Part model, mm, in its own coordinate system. Face numbers are marked on the shaded views. A direction names the side the tool comes from. Round coordinates to 2 decimals unless told otherwise and drop trailing zeros. Loops run counter-clockwise (first coordinate to the right, second up) from the corner with the lowest first, then second, coordinate; pieces in that order, holes last. Notation, with made-up numbers: M 56,54.25 L 72,54.25 A21 cw 72,92.25 Z; hole C 89,34 d2. An arc over 180 degrees is marked long. Put each result on its own line as item: value. Start each with the question number.
1) Drop a flat-ended pin along its axis: pin 1 Ø10 at (x, y) = (82, -842) entering from -Z. Give the stop position or say it passes through.
2) Slice it at C-C on z = 17. Give the cut face in (x, y).
3) Probe line 1 along X through (y, z) = (-778, 1.15); line 2 along X through (y, z) = (-776, 12); line 3 along Z through (x, y) = (9.5, -523.5). List the from-to ranges inside material, lowest first.
4) Pull direction X, two halves, no side cores. Call the marked faces 3 and 4: +X half, -X half, draft (parallel to the pull), parting line (faces both ways), or undercut.
5) Slice it at A-A on y = -115. Give the cut face in (x, z), then the cut area to 3 significant figures.
6) Slice it at B-B on x = 50. Give the cut face in (y, z).
7) Which spindle directions (+Z, -Z, +X, -X, +Y, -Y) get a long thin tool onto all of the face, cutting with end or side? Do the marked faces 1 and 2. Say none if no direction does.
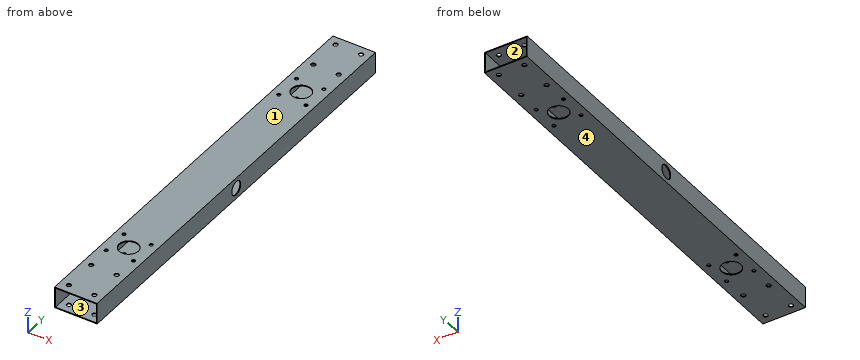
```python
from build123d import *

# Parameters (mm, degrees)
F0_W     = 100
F0_H     = 50
F0_W_2   = 96
F0_H_2   = 46
F1_DEPTH = 1000
F2_R     = 22.5
F3_DEPTH = 50.001
F5_D     = 8.5
F6_D     = 10.5
F7_R     = 16
F8_DEPTH = 100.001


with BuildPart() as f1:
    # F0 (on Front) → F1 (new body)
    with BuildSketch(Plane.XZ):
        with Locations((50, 25)):
            Rectangle(F0_W, F0_H)
        with Locations((50, 25)):
            Rectangle(F0_W_2, F0_H_2, mode=Mode.SUBTRACT)
    extrude(amount=F1_DEPTH)

    # F2 (on face) → F3 (cut, through all)
    with BuildSketch(Plane.XY.offset(50)):
        with Locations((50, -810)):
            Circle(F2_R)
        with Locations((50, -190)):
            Circle(F2_R)
    extrude(amount=-F3_DEPTH, mode=Mode.SUBTRACT)

    # F5 (through all)
    with Locations(Plane.XY.offset(50)):
        with Locations((18, -842), (18, -778), (82, -778), (82, -842), (18, -222), (18, -158), (82, -158), (82, -222)):
            Hole(F5_D / 2)

    # F6 (through all)
    with Locations(Plane.XY.offset(50)):
        with Locations((20, -101), (20, -21), (80, -21), (80, -101), (20, -899), (20, -979), (80, -979), (80, -899)):
            Hole(F6_D / 2)

    # F7 (on face) → F8 (cut, through all)
    with BuildSketch(Plane.YZ.offset(100)):
        with Locations((-500, 25)):
            Circle(F7_R)
    extrude(amount=-F8_DEPTH, mode=Mode.SUBTRACT)


solid = f1.part
```
Recorded:
1. pin 1: stops at z = 0
2. outline: M 0,-1000 L 2,-1000 L 2,-513.86 L 0,-513.86 Z; M 0,-486.14 L 2,-486.14 L 2,0 L 0,0 Z; M 98,-1000 L 100,-1000 L 100,-513.86 L 98,-513.86 Z; M 98,-486.14 L 100,-486.14 L 100,0 L 98,0 Z
3. line 1: x = 0 to 13.75, 22.25 to 77.75, 86.25 to 100
3. line 2: x = 0 to 2, 98 to 100
3. line 3: z = 0 to 2, 48 to 50
4. face 3: undercut
4. face 4: draft
5. outline: M 0,0 L 100,0 L 100,50 L 0,50 Z; hole M 2,2 L 98,2 L 98,48 L 2,48 Z
5. area: 584 mm2
6. outline: M -1000,0 L -832.5,0 L -832.5,2 L -1000,2 Z; M -1000,48 L -832.5,48 L -832.5,50 L -1000,50 Z; M -787.5,0 L -212.5,0 L -212.5,2 L -787.5,2 Z; M -787.5,48 L -212.5,48 L -212.5,50 L -787.5,50 Z; M -167.5,0 L 0,0 L 0,2 L -167.5,2 Z; M -167.5,48 L 0,48 L 0,50 L -167.5,50 Z
7. face 1: +Z, +X, -X, +Y, -Y
7. face 2: +Y, -Y
